Check sheet for the modelled part. Datum: model origin and axes. Units: mm. Face numbers are marked on the shaded views. A direction names the side the tool comes from. Round coordinates to 2 decimals unless told otherwise and drop trailing zeros. Write each loop counter-clockwise with the first axis right and the second up, starting at its lowest first coordinate (ties: lowest second). Pieces come first, ordered by that corner, then holes. Notation, with made-up numbers: (-10, 79) -> (49, 79) arc R27 cw to (49, 105) -> close; hole circle Ø6 at (38, 37.25). An arc over 180 degrees is marked (long way). Answer as a JSON object with one key per item and string values. Group by question number.
```python
from build123d import *

# Parameters (mm, degrees)
SKETCH1_W                = 33
SKETCH1_H                = 33
SKETCH1_R                = 1.824627508
SKETCH1_W_2              = 15
SKETCH1_H_2              = 4
BOSS_EXTRUDE1_DEPTH      = 2
SKETCH2_W                = 36.501337607
SKETCH2_H                = 33
SKETCH2_R                = 1.5
BOSS_EXTRUDE2_DEPTH      = 2
BOSS_EXTRUDE3_DEPTH      = 2
BOSS_EXTRUDE3_DEPTH_BACK = 15
SKETCH1_3_W              = 2
SKETCH1_3_H              = 33
FILLET1_R                = 7
FILLET2_R                = 16.5
FILLET3_R                = 3


# Some blends are built 0.0001 mm under size
with BuildPart() as part:
    # Sketch1 → Boss-Extrude1 (new body)
    with BuildSketch(Plane(origin=(0, 0, 0), x_dir=(1, 0, 0), z_dir=(0, 1, 0))):
        Rectangle(SKETCH1_W, SKETCH1_H)
        with Locations(Location((-13, -13, 0), (0, 0, 270))):
            Circle(SKETCH1_R, mode=Mode.SUBTRACT)
        with Locations(Location((13, -13, 0), (0, 0, 270))):
            Circle(SKETCH1_R, mode=Mode.SUBTRACT)
        with Locations(Location((13, 13, 0), (0, 0, 270))):
            Circle(SKETCH1_R, mode=Mode.SUBTRACT)
        with Locations(Location((-13, 13, 0), (0, 0, 270))):
            Circle(SKETCH1_R, mode=Mode.SUBTRACT)
        with Locations((0, 13)):
            Rectangle(SKETCH1_W_2, SKETCH1_H_2, mode=Mode.SUBTRACT)
        with Locations((0, -13)):
            Rectangle(SKETCH1_W_2, SKETCH1_H_2, mode=Mode.SUBTRACT)
    extrude(amount=BOSS_EXTRUDE1_DEPTH)



with BuildPart() as body_2:
    # Sketch2 → Boss-Extrude2 (new body)
    with BuildSketch(Plane(origin=(0, -15, 0), x_dir=(1, 0, 0), z_dir=(0, 1, 0))):
        with Locations((34.750668804, 0)):
            Rectangle(SKETCH2_W, SKETCH2_H)
        with Locations(Location((34.210179074, 10, 0), (0, 0, 270))):
            Circle(SKETCH2_R, mode=Mode.SUBTRACT)
        with Locations(Location((49.210179074, 0, 0), (0, 0, 270))):
            Circle(SKETCH2_R, mode=Mode.SUBTRACT)
        with Locations(Location((34.210179074, -10, 0), (0, 0, 270))):
            Circle(SKETCH2_R, mode=Mode.SUBTRACT)
    extrude(amount=BOSS_EXTRUDE2_DEPTH)


with BuildPart() as part_1:
    add(part.part)

    add(body_2.part)  # Boss-Extrude3 merges body 2
    # Sketch1<3> → Boss-Extrude3 (add, two sides: drawn at the far end of the back side and taken through both)
    with BuildSketch(Plane(origin=(0, 0, 0), x_dir=(1, 0, 0), z_dir=(0, 1, 0)).offset(-BOSS_EXTRUDE3_DEPTH_BACK)):
        with Locations((17.5, 0)):
            Rectangle(SKETCH1_3_W, SKETCH1_3_H)
    extrude(amount=BOSS_EXTRUDE3_DEPTH + BOSS_EXTRUDE3_DEPTH_BACK)

    # Fillet1
    # the kernel refuses this fillet: 7 mm, written as the material it adds along each edge
    with BuildSketch(Plane(origin=(16.5, 0, -16.5), x_dir=(0, -1, 0), z_dir=(0, 0, 1))) as fillet1_piece_1_section:
        with BuildLine():
            CenterArc((FILLET1_R, -FILLET1_R), FILLET1_R, 90, 90)
            Line((0, -FILLET1_R), (0, 0))
            Line((0, 0), (FILLET1_R, 0))
        make_face()
    fillet1_piece_1 = extrude(amount=33, mode=Mode.PRIVATE)
    fillet1_piece_1 = fillet1_piece_1 - Plane(origin=(13, -1.648536781, -13), x_dir=(0, 0, 1), z_dir=(0, -1, 0)) * Cylinder(1.824627508, 94, mode=Mode.PRIVATE)
    fillet1_piece_1 = fillet1_piece_1 - Plane(origin=(13, -1.648536781, 13), x_dir=(0, 0, 1), z_dir=(0, -1, 0)) * Cylinder(1.824627508, 94, mode=Mode.PRIVATE)
    add(fillet1_piece_1)
    with BuildSketch(Plane(origin=(18.5, -13, 16.5), x_dir=(0, 1, 0), z_dir=(0, 0, -1))) as fillet1_piece_2:
        with BuildLine():
            CenterArc((FILLET1_R, FILLET1_R), FILLET1_R, 180, 90)
            Line((0, FILLET1_R), (0, 0))
            Line((0, 0), (FILLET1_R, 0))
        make_face()
    extrude(amount=33)
    # the kernel refuses this fillet: 7 mm, written as the material it takes off along each edge
    with BuildSketch(Plane(origin=(18.5, 2, 34), x_dir=(-1, 0, 0), z_dir=(0, 0, -1)), Plane(origin=(16.5, -15, 34), x_dir=(1, 0, 0), z_dir=(0, 0, -1))) as fillet1_2_piece_1:
        with BuildLine():
            CenterArc((FILLET1_R, -FILLET1_R), FILLET1_R, 90, 90)
            Line((0, -FILLET1_R), (0, 0))
            Line((0, 0), (FILLET1_R, 0))
        make_face()
    extrude(amount=68, mode=Mode.SUBTRACT)

    # Fillet2
    fillet2_edges = [part_1.edges().sort_by_distance(p)[0] for p in [
        (53.001337607, -14, -16.5),
        (53.001337607, -14, 16.5),
    ]]
    fillet(fillet2_edges, radius=FILLET2_R - 0.0001)  # a hair under: the kernel refuses the full size

    # Fillet3
    fillet3_edges = [part_1.edges().sort_by_distance(p)[0] for p in [
        (-16.5, 1, 16.5),
        (-16.5, 1, -16.5),
    ]]
    fillet(fillet3_edges, radius=FILLET3_R)


solid = part_1.part
```
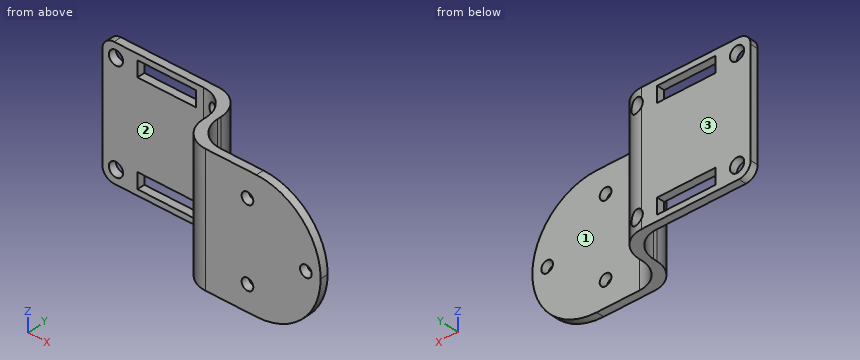
(1) Section check D-D on x = 28. Record the cut outline in (y, z).
(2) Scan lines: line 1 along Z through (x, y) = (-5.5, 0.25); line 2 along Z through (x, y) = (13, 0.3); line 3 along Y through (x, z) = (36, -1.5). Record each from-to range of solid material in increasing order.
(3) Access from +Z, -Z, +X, -X, +Y, -Y to the whole of each face (thin tool, end or side, straight path). Record for the marked faces 1, 2 and 3.
(4) Section check A-A on x = 6.5. Record the cut outline in (y, z).
(5) Section check B-B on x = 35. Record the cut outline in (y, z), then the cut area to 3 significant figures.
(6) Go/stop test with flat-tipped pins: pin 1 Ø5 at (x, z) = (10.5, 7) entering from -Y; pin 2 Ø0.5 at (y, z) = (-7.5, -0.5) entering from -X; pin 3 Ø6 at (x, z) = (-13, -13) entering from -Y. Record where each tip stops, or that it passes through.
(7) Section check C-C on z = 4. Record the cut outline in (x, y).
Data:
{
 "1": {"outline": "(-15, -16.5) -> (-13, -16.5) -> (-13, 16.5) -> (-15, 16.5) -> close"},
 "2": {"line 1": "z = -16.5 to -15, -11 to 11, 15 to 16.5", "line 2": "z = -16.5 to -14.82, -11.18 to 11.18, 14.82 to 16.5", "line 3": "y = -15 to -13"},
 "3": {"face 1": "+Z, -Z, +X, +Y", "face 2": "+Z, -Z, -X, -Y", "face 3": "+Z, -Z, +X, -X, +Y"},
 "4": {"outline": "(0, -16.5) -> (2, -16.5) -> (2, -15) -> (0, -15) -> close; (0, -11) -> (2, -11) -> (2, 11) -> (0, 11) -> close; (0, 15) -> (2, 15) -> (2, 16.5) -> (0, 16.5) -> close"},
 "5": {"outline": "(-15, -16.5) -> (-13, -16.5) -> (-13, -11.28) -> (-15, -11.28) -> close; (-15, -8.72) -> (-13, -8.72) -> (-13, 8.72) -> (-15, 8.72) -> close; (-15, 11.28) -> (-13, 11.28) -> (-13, 16.5) -> (-15, 16.5) -> close", "area": "55.8 mm²"},
 "6": {"pin 1": "stops at y = -0.94", "pin 2": "stops at x = 16.5", "pin 3": "stops at y = 0"},
 "7": {"outline": "(-16.5, 0) -> (9.5, 0) arc R7 cw to (16.5, -7) -> (16.5, -8) arc R7 ccw to (23.5, -15) -> (52.51, -15) -> (52.51, -13) -> (25.5, -13) arc R7 cw to (18.5, -6) -> (18.5, -5) arc R7 ccw to (11.5, 2) -> (-16.5, 2) -> close"}
}
